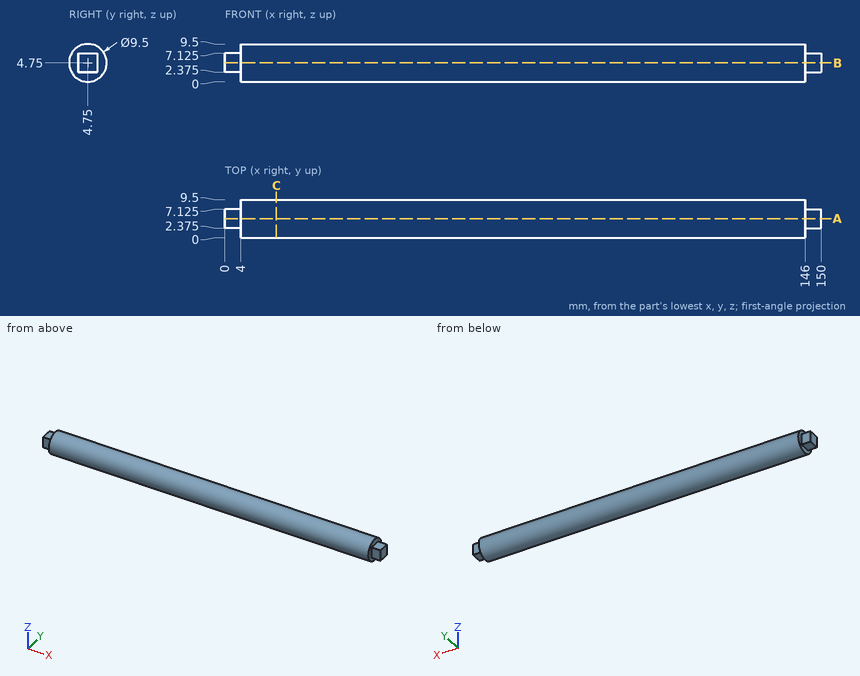
Job drawing, mm, ordinate dimensions from the low corner. One solid piece. Coordinates: 2 decimals unless noted, no trailing zeros. Order: outer loops, then holes, each group sorted by start corner. A loop starts at its lowest first (then second) coordinate and runs counter-clockwise, first axis right, second up. Notation, with made-up numbers: (4, 47) - (28, 47) arc R14 cw to (28, 74) - close; hole circle Ø7 at (2, 19.25). An arc over 180 degrees is marked (long way). Write each question's results on one line, items separated by ' | '. Start each with the question number.
Item 1: Band-saw the part on C-C on x = 13. Write the cut outline in (y, z).
Item 2: Wall check: probe 1 along X at (y, z) = (6, 1.25); probe 2 along Z at (x, y) = (30.5, 4.5). Give the ranges that are in metal, low to high. Write a range as [from, to].
Item 3: Band-saw the part on A-A on y = 4.75. Write the cut outline in (x, z) (3 decimals).
Item 4: Flat gauge pins, fed straight in: pin 1 (4 mm diameter, centred on x = 112.5, y = 7.5, fed in from -Z); pin 2 (1.2 mm diameter, centred on x = 2, y = 4, fed in from +Z) (3 decimals); pin 3 (1.2 mm diameter, centred on x = 1.5, z = 5.5, fed in from +Y) (3 decimals). Where does each tip first touch, or does it go through?
Numbers:
1) outline: circle Ø9.5 at (4.75, 4.75)
2) probe 1: [4, 146] | probe 2: [0.01, 9.49]
3) outline: (0, 2.375) - (4, 2.375) - (4, 0) - (146, 0) - (146, 2.375) - (150, 2.375) - (150, 7.125) - (146, 7.125) - (146, 9.5) - (4, 9.5) - (4, 7.125) - (0, 7.125) - close
4) pin 1: z = 0.06 | pin 2: z = 7.125 | pin 3: y = 7.125
